Design review of the part built by this model. Coordinates are the model's own, in mm. A direction names the side the tool comes from. Give positions to 0.01 mm unless a question says otherwise; leave off trailing zeros. Loops run counter-clockwise (first coordinate to the right, second up) from the corner with the lowest first, then second, coordinate; pieces in that order, holes last.
from build123d import *

# Parameters (mm, degrees)
BLANKSKE_W        = 80
BLANKSKE_H        = 10.8
BLANK_DEPTH       = 7.4
TOOTHCUTSIM_DEPTH = 82.064172111
TEETHCUTS_COUNT   = 33
TEETHCUTS_PITCH   = 2.51327412
SKETCH_1_R        = 2
EXTRUDE_1_DEPTH   = 10


with BuildPart() as part:
    # BlankSke → Blank (new body)
    with BuildSketch(Plane.XY):
        with Locations((40, 5.4)):
            Rectangle(BLANKSKE_W, BLANKSKE_H)
    extrude(amount=-BLANK_DEPTH)

    # TooCutSkeSim → ToothCutSim (cut, through all)
    with BuildSketch(Plane.XY):
        Polygon((0.354348296, 9), (-0.354348296, 9), (-1.018739561, 10.8254), (1.018739561, 10.8254), align=None)
    toothcutsim = extrude(amount=-TOOTHCUTSIM_DEPTH, mode=Mode.SUBTRACT)

    # TeethCuts: ToothCutSim ×33
    with Locations(*[(i * TEETHCUTS_PITCH, 0, 0) for i in range(1, TEETHCUTS_COUNT)]):
        add(toothcutsim, mode=Mode.SUBTRACT)

    # 草图1 → 凸台-拉伸1 (add)
    with BuildSketch(Plane.ZY):
        with Locations((-3.7, 5.4)):
            Circle(SKETCH_1_R)
    extrude(amount=EXTRUDE_1_DEPTH)


solid = part.part
Q1. Wall thickness on line 1 (Y direction, x = 57.5, z = -1.5); line 2 (X direction, y = 2, z = -5.5); line 3 (Z direction, x = -4.5, y = 5): over which ranges is each line inside the solid? List them lowest first.
Results:
line 1: y = 0 to 9
line 2: x = 0 to 80
line 3: z = -5.66 to -1.74
Q2. Tool access review of faces 4 (the face through (49.588, 9.887, -3.648)), 5 (the face through (0, 3, -4)): name each direction out of +Z, -Z, +X, -X, +Y, -Y from which nothing blocks a thin tool from reaching the whole face with its end or side.
Results:
face 4: +Z, -Z, +Y
face 5: -X
Q3. Take a section at A-A (y = 5.4). Give the boundary of the cut face in (x, z).
Results:
outline: (-10, -5.7) - (0, -5.7) - (0, -7.4) - (80, -7.4) - (80, 0) - (0, 0) - (0, -1.7) - (-10, -1.7) - close
Q4. Draft analysis for pull direction X (two halves, no side actions). For faces 1 (the face through (39, 5, 0)), 2 (the face through (71.058, 9.913, -3.648)), 3 (the face through (80, 5, -4)), state which applies: pulls with the +X half, pulls with the -X half, needs draft (parallel to the pull), parting line crosses it, or undercut.
Results:
face 1: needs draft
face 2: undercut
face 3: pulls with the +X half
Q5. Insertion check: pin 1 (1 mm diameter, centred on y = 8.5, z = -2.5, fed in from -X). The pin has a flat end and moves straight along its axis. Give the tip position at first contact, or say it passes through.
Results:
pin 1: stops at x = 0
